Part model, mm, in its own coordinate system. A direction names the side the tool comes from. Give positions to 0.01 mm unless a question says otherwise; leave off trailing zeros. Order: outer loops, then holes, each group sorted by start corner. A loop starts at its lowest first (then second) coordinate and runs counter-clockwise, first axis right, second up. Notation, with made-up numbers: M 63.5,-24.5 L 69.5,-24.5 A13 cw 69.5,-20.5 Z; hole C 89,67.5 d1. An arc over 180 degrees is marked long. One line per question, with ' | ' between items.
Autodesk Inventor part; units mm, degrees
ref_plane "YZ Plane" through (0, 0, 0) normal (1, 0, 0) x (0, 1, 0)
ref_plane "XZ Plane" through (0, 0, 0) normal (0, 1, 0) x (-1, 0, 0)
ref_plane "XY Plane" through (0, 0, 0) normal (0, 0, 1) x (1, 0, 0)
sketch "Sketch6" plane through (0, 0, 0) normal (0, 0, 1) x (1, 0, 0)
  circle A0 centre (0, 0) radius 9
  circle A1 centre (0, 0) radius 14
  dimension "d20" = 18
  dimension "d21" = 28
extrude "Extrusion4" add sketch "Sketch6" along normal blind 35
ref_plane "Work Plane2" through (0, 0, 17.5) normal (0, 0, 1) x (1, 0, 0)
sketch "Sketch8" plane through (0, 0, 17.5) normal (0, 0, 1) x (1, 0, 0)
  line L0 (0, 0) -> (0, 26)
  line L1 (0, 26) -> (-9.5, 26)
  line L2 (-9.5, 26) -> (-9.5, 21.5)
  line L3 (-9.5, 21.5) -> (0, 21.5)
  line L4 (0, 21.5) -> (0, 26)
  line L5 (0, 21.5) -> (-9.5, 21.5)
  line L6 (-9.5, 21.5) -> (-9.5, 18.5)
  line L7 (-9.5, 18.5) -> (0, 18.5)
  line L8 (0, 18.5) -> (0, 21.5)
  line L9 (9.5, 21.5) -> (0, 21.5)
  line L10 (9.5, 21.5) -> (9.5, 18.5)
  line L11 (9.5, 18.5) -> (0, 18.5)
  dimension "d28" = 26
  dimension "d29" = 9.5
  dimension "d30" = 4.5
  dimension "d32" = 3
revolve "Revolution1" add sketch "Sketch8" angle 360 about axis through (0, 26, 17.5) along (-1, 0, 0) contours L7 L6 L3 L0 | L0 L9 L10 L11
sketch "Sketch10" plane through (0, 0, 17.5) normal (0, 0, 1) x (1, 0, 0)
  circle A0 centre (0, 0) radius 14
  line L0 (-14, 0) -> (-9.5, 19)
  line L1 (-9.5, 19) -> (0, 19)
  line L2 (-9.5, 33.5) -> (-9.5, 18.5)
  line L3 (0, 19) -> (0, 0)
  line L4 (14, 0) -> (9.5, 19)
  line L5 (9.5, 19) -> (0, 19)
  point P0 (-12.5128, 6.2793)
  point P1 (12.5128, 6.2793)
  dimension "d35" = 19
  dimension "d36" = 9.5
extrude "Extrusion6" add sketch "Sketch10" along normal blind 2.5 contours L0 L1 L3 A0 | A0 L3 L5 L4
mirror "Mirror2" about plane through (0, 0, 17.5) normal (0, 0, 1) of "Extrusion6"
ref_plane "Work Plane3" through (0, 59.1111, 15) normal (-1, 0, 0) x (0, 0, 1)
sketch "Sketch11" plane through (0, 59.1111, 15) normal (-1, 0, 0) x (0, 0, 1)
  arc A0 (5, -40.1822) -> (0, -40.1822) centre (2.5, -33.1111) ccw
  line L0 (-4.9336, -34.1072) -> (-15, -45.1111)
  line L1 (-15, -45.1111) -> (20, -45.1111)
  circle A1 centre (2.5, -33.1111) radius 7.5
  line L2 (2.5, -33.1111) -> (2.5, -59.6944)
  line L3 (10, -34.1161) -> (20, -45.1111)
  point P0 (-15, -59.1111)
  point P1 (10, -33.1111)
  point P2 (2.5, -45.1111)
  point P3 (2.5, -40.6111)
extrude "Extrusion9" add sketch "Sketch11" along normal blind 2.5 contours L2 L1 L0 A0 A1
mirror "Mirror5" about plane through (0, 59.1111, 15) normal (-1, 0, 0) of "Extrusion9"
mirror "Mirror6" about plane through (0, 0, 17.5) normal (0, 0, 1) of "Extrusion9", "Mirror5"
sketch "Sketch13" plane through (2.5, 25.0039, 10.0664) normal (0, 0.675, -0.7378) x (-1, 0, 0)
  line L0 (0, 0) -> (5, 0)
  line L1 (0, 0) -> (5, 0)
  line L2 (5, 0) -> (5, 11.3934)
  line L3 (5, 11.3934) -> (0, 11.3934)
  line L4 (0, 11.3934) -> (0, 0)
  line L5 (0, 11.3934) -> (5, 0)
  line L6 (0, 0) -> (5, 11.3934)
  line L7 (2.5, -1.4142) -> (2.5, 8.7105)
  circle A0 centre (2.5, 5.6967) radius 2.0284
  point P0 (2.5, -25.2434)
extrude "Extrusion10" add sketch "Sketch13" along normal blind 15 contours A0 L5 L6 | L6 L7 A0 | L7 L5 A0 | A0 L7 L5 | L6 A0 L5 | L7 A0 L6
mirror "Mirror7" about plane through (0, 0, 17.5) normal (0, 0, 1) of "Extrusion10"
1. Mould opens along Z. For faces 1 (the flat face through (-0.04, 19.42, 4.96)), 2 (the flat face through (-2.5, 17, 26)), 3 (the cylindrical face through (0.13, 26.59, 13.04)) say: released by +Z, released by -Z, zero draft, split by the parting line, or undercut.
Worked out:
face 1: released by -Z | face 2: zero draft | face 3: undercut
2. Slice it at B-B on y = 26. Give the cut face in (x, z), then the cut area to 3 significant figures.
Worked out:
outline: M -9.5,10 L 9.5,10 L 9.5,13 L -9.5,13 Z; M -9.5,22 L 9.5,22 L 9.5,25 L -9.5,25 Z | area: 114 mm2
3. Drop flat-ended pins along their axis: pin 1 (5 mm diameter, centred on x = 9.5, z = 24.5, fed in from +Y); pin 2 (1.5 mm diameter, centred on x = 1, z = 4, fed in from +Y); pin 3 (10 mm diameter, centred on x = 6, z = 21.5, fed in from -Y). Give the stop position or say it passes through.
Worked out:
pin 1: stops at y = 32 | pin 2: stops at y = 40.81 | pin 3: stops at y = -13.96
4. Probe L1, parallel to Y at x = 5.25, z = 23; L2, parallel to Y at x = 6.25, z = 14.5; L3, parallel to Y at x = -2.75, z = 19.5. List the from-to ranges inside material, lowest first. Write a range as from..to.
Worked out:
L1: y = -12.98..-7.31, 7.31..12.98, 20.9..31.1 | L2: y = -12.53..-6.48, 6.48..12.53, 19.13..22.65, 29.35..32.87 | L3: y = -13.73..-8.57, 8.57..21.97, 30.03..33.23
5. Slice it at C-C on x = -5.5. Give the cut face in (y, z), then the cut area to 3 significant figures.
Worked out:
outline: M -12.87,0 L -7.12,0 L -7.12,35 L -12.87,35 Z; M 7.12,0 L 12.87,0 L 12.87,15 L 18.93,15 A7.5 ccw long 18.93,20 L 12.87,20 L 12.87,35 L 7.12,35 Z; hole C 26,17.5 d9 | area: 544 mm2
6. Tool access for faces 4 (the flat face through (2.5, 17, 26)), 5 (the flat face through (-9.5, 21, 18)), 6 (the flat face through (2.5, 17, 9)), 7 (the flat face through (-2.5, 17, 9)): list every direction of +Z, -Z, +X, -X, +Y, -Y with a clear straight run to the whole face (end or side of a thin tool).
Worked out:
face 4: +Z, +X | face 5: +Z, -Z, -X, +Y | face 6: -Z, +X | face 7: -Z, -X
7. Slice it at A-A on z = 17.5. Give the cut face in (x, y), then the cut area to 3 significant figures.
Worked out:
outline: M -12.51,6.28 A14 ccw long 12.51,6.28 L 9.5,19 L 9.5,21.5 L -9.5,21.5 L -9.5,19 Z; M -9.5,30.5 L 9.5,30.5 L 9.5,33.5 L -9.5,33.5 Z; hole C 0,0 d18 | area: 608 mm2
